Autodesk Inventor part; units mm, degrees
ref_plane "YZ Plane" through (0, 0, 0) normal (1, 0, 0) x (0, 1, 0)
ref_plane "XZ Plane" through (0, 0, 0) normal (0, 1, 0) x (-1, 0, 0)
ref_plane "XY Plane" through (0, 0, 0) normal (0, 0, 1) x (1, 0, 0)
sketch "Sketch1" plane through (0, 0, 0) normal (0, 0, 1) x (1, 0, 0)
  line L0 (11.7695, 33.9618) -> (11.7695, -67.6382)
  line L1 (100.6695, 33.9618) -> (100.6695, -67.6382)
  line L2 (18.1195, 40.3118) -> (94.3195, 40.3118)
  line L3 (24.4695, -80.3382) -> (87.9695, -80.3382)
  arc A0 (11.7695, -67.6382) -> (24.4695, -80.3382) centre (24.4695, -67.6382) ccw
  arc A1 (87.9695, -80.3382) -> (100.6695, -67.6382) centre (87.9695, -67.6382) ccw
  arc A2 (100.6695, 33.9618) -> (94.3195, 40.3118) centre (94.3195, 33.9618) ccw
  arc A3 (18.1195, 40.3118) -> (11.7695, 33.9618) centre (18.1195, 33.9618) ccw
  point P0 (0, 0)
  dimension "d0" = 12.7
  dimension "d1" = 6.35
  dimension "d2" = 120.65
  dimension "d3" = 88.9
extrude "Extrusion1" add sketch "Sketch1" along normal blind 4.7625
sketch "Sketch2" plane through (0, 0, 4.7625) normal (0, 0, 1) x (1, 0, 0)
  line L0 (11.7695, -67.6382) -> (11.7695, 33.9618)
  line L1 (100.6695, 33.9618) -> (100.6695, -67.6382)
  line L2 (18.1195, 40.3118) -> (94.3195, 40.3118)
  line L3 (17.7131, 34.3682) -> (94.7259, 34.3682)
  line L4 (94.7259, 34.3682) -> (94.7259, -29.6652)
  line L5 (94.7259, -29.6652) -> (17.7131, -29.6652)
  line L6 (17.7131, -29.6652) -> (17.7131, 34.3682)
  point P0 (0, 0)
  dimension "d6" = 5.9436
  dimension "d7" = 5.9436
  dimension "d8" = 5.9436
  dimension "d9" = 64.0334
  dimension "d54" = 77.0128
extrude "Extrusion2" cut sketch "Sketch2" against normal through all
sketch "Sketch3" plane through (0, 0, 4.7625) normal (0, 0, 1) x (1, 0, 0)
  line L0 (17.7131, -29.6652) -> (17.7131, 34.3682)
  line L1 (94.7259, 34.3682) -> (94.7259, -29.6652)
  line L2 (94.7259, -29.6652) -> (17.7131, -29.6652)
  line L3 (30.4131, -29.6652) -> (30.4131, -34.7452)
  line L4 (30.4131, -34.7452) -> (82.0259, -34.7452)
  line L5 (82.0259, -34.7452) -> (82.0259, -29.6652)
  point P0 (0, 0)
  dimension "d13" = 12.7
  dimension "d14" = 12.7
  dimension "d15" = 5.08
extrude "Extrusion3" cut sketch "Sketch3" against normal through all
sketch "Sketch4" plane through (0, 0, 4.7625) normal (0, 0, 1) x (1, 0, 0)
  line L0 (17.7131, -29.6652) -> (17.7131, 34.3682)
  line L1 (94.7259, 34.3682) -> (94.7259, -29.6652)
  line L2 (82.0259, -34.7452) -> (30.4131, -34.7452)
  arc A0 (11.7695, -67.6382) -> (24.4695, -80.3382) centre (24.4695, -67.6382) ccw
  line L3 (87.9695, -80.3382) -> (24.4695, -80.3382)
  arc A1 (87.9695, -80.3382) -> (100.6695, -67.6382) centre (87.9695, -67.6382) ccw
  line L4 (24.4695, -73.9882) -> (87.9695, -73.9882)
  line L5 (17.7131, -32.8402) -> (17.7131, -67.2318)
  line L6 (94.7259, -32.8402) -> (94.7259, -67.2318)
  arc A2 (17.7131, -67.2318) -> (24.4695, -73.9882) centre (24.4695, -67.2318) ccw
  arc A3 (87.9695, -73.9882) -> (94.7259, -67.2318) centre (87.9695, -67.2318) ccw
  line L7 (30.4131, -34.7452) -> (30.4131, -29.6652)
  line L8 (30.4131, -29.6652) -> (17.7131, -29.6652)
  line L9 (82.0259, -29.6652) -> (82.0259, -34.7452)
  line L10 (30.4131, -32.8402) -> (17.7131, -32.8402)
  line L11 (82.0259, -32.8402) -> (94.7259, -32.8402)
  point P0 (0, 0)
  dimension "d18" = 6.35
  dimension "d21" = 3.175
extrude "Extrusion4" cut sketch "Sketch4" against normal through all
sketch "Sketch6" plane through (0, 0, 4.7625) normal (0, 0, 1) x (1, 0, 0)
  line L0 (87.9695, -80.3382) -> (24.4695, -80.3382)
  circle A0 centre (37.1695, 37.1876) radius 1.27
  circle A1 centre (75.2695, 37.1876) radius 1.27
  circle A2 centre (37.1695, -77.214) radius 1.27
  circle A3 centre (75.2695, -77.214) radius 1.27
  circle A4 centre (14.8937, 21.2618) radius 1.27
  circle A5 centre (14.8937, -16.8382) radius 1.27
  circle A6 centre (97.5453, 21.2618) radius 1.27
  circle A7 centre (97.5453, -16.8382) radius 1.27
  line L1 (18.1195, 40.3118) -> (94.3195, 40.3118)
  line L2 (11.7695, -67.6382) -> (11.7695, 33.9618)
  line L3 (100.6695, 33.9618) -> (100.6695, -67.6382)
  point P0 (0, 0)
  dimension "d35" = 3.1242
  dimension "d36" = 3.1242
  dimension "d37" = 3.1242
  dimension "d38" = 3.1242
  dimension "d39" = 2.54
  dimension "d40" = 25.4
  dimension "d41" = 19.05
  dimension "d42" = 25.4
  dimension "d43" = 38.1
extrude "Extrusion5" cut sketch "Sketch6" against normal through all
sketch "Sketch7" plane through (0, 0, 4.7625) normal (0, 0, 1) x (1, 0, 0)
  circle A0 centre (97.5453, -16.8382) radius 1.27
  circle A1 centre (97.5453, 21.2618) radius 1.27
  circle A2 centre (14.8937, -16.8382) radius 1.27
  circle A3 centre (14.8937, 21.2618) radius 1.27
  circle A4 centre (75.2695, -77.214) radius 1.27
  circle A5 centre (37.1695, -77.214) radius 1.27
  circle A6 centre (75.2695, 37.1876) radius 1.27
  circle A7 centre (37.1695, 37.1876) radius 1.27
  line L0 (17.7131, -32.8402) -> (30.4131, -32.8402)
  line L1 (30.4131, -32.8402) -> (30.4131, -29.6652)
  line L2 (30.4131, -29.6652) -> (17.7131, -29.6652)
  line L3 (17.7131, -29.6652) -> (17.7131, 34.3682)
  line L4 (17.7131, 34.3682) -> (94.7259, 34.3682)
  line L5 (94.7259, 34.3682) -> (94.7259, -29.6652)
  line L6 (94.7259, -29.6652) -> (82.0259, -29.6652)
  line L7 (82.0259, -29.6652) -> (82.0259, -32.8402)
  line L8 (82.0259, -32.8402) -> (94.7259, -32.8402)
  line L9 (94.7259, -32.8402) -> (94.7259, -67.2318)
  arc A8 (87.9695, -73.9882) -> (94.7259, -67.2318) centre (87.9695, -67.2318) ccw
  line L10 (87.9695, -73.9882) -> (24.4695, -73.9882)
  arc A9 (17.7131, -67.2318) -> (24.4695, -73.9882) centre (24.4695, -67.2318) ccw
  line L11 (17.7131, -67.2318) -> (17.7131, -32.8402)
  arc A10 (18.1195, 40.3118) -> (11.7695, 33.9618) centre (18.1195, 33.9618) ccw
  line L12 (11.7695, -67.6382) -> (11.7695, 33.9618)
  arc A11 (11.7695, -67.6382) -> (24.4695, -80.3382) centre (24.4695, -67.6382) ccw
  line L13 (87.9695, -80.3382) -> (24.4695, -80.3382)
  arc A12 (87.9695, -80.3382) -> (100.6695, -67.6382) centre (87.9695, -67.6382) ccw
  line L14 (100.6695, 33.9618) -> (100.6695, -67.6382)
  arc A13 (100.6695, 33.9618) -> (94.3195, 40.3118) centre (94.3195, 33.9618) ccw
  line L15 (18.1195, 40.3118) -> (94.3195, 40.3118)
  line L16 (11.7695, -61.2882) -> (30.8195, -80.3382)
  line L17 (81.6195, -80.3382) -> (100.6695, -61.2882)
  point P0 (0, 0)
  dimension "d46" = 6.35
  dimension "d47" = 5.9436
  dimension "d48" = 82.9564
  dimension "d49" = 13.1064
  dimension "d50" = 12.7
  dimension "d51" = 19.05
  dimension "d52" = 19.05
  dimension "d53" = 69.85
properties part number "lcd_spacer"
Here's how the part is built. I have some questions about the finished solid (model axes, mm). A direction names the side the tool comes from. Give positions to 0.01 mm unless a question says otherwise; leave off trailing zeros. Order: outer loops, then holes, each group sorted by start corner. A loop starts at its lowest first (then second) coordinate and runs counter-clockwise, first axis right, second up. Notation, with made-up numbers: (22, -12.5) -> (30, -12.5) arc R24 ccw to (30, 11.5) -> close; hole circle Ø7 at (-2, -12). An arc over 180 degrees is marked (long way). Use CSV: the item, a comma, the result in double quotes. Start each with the question number.
Item 1: Suppose I cut it at C-C (x = 44.5). List the corners of the cut face in (y, z) for me.
Item 2: Thinking about a two-plate mould opening in Y: for faces 1 (the cylindrical face through (75.104, -75.955, 2.415)), 2 (the flat face through (56, -73.988, 2)), 3 (the flat face through (96, -20, 4.762)), 4 (the cylindrical face through (97.048, -76.519, 2.348)), which applies, pulls with the +Y half, pulls with the -Y half, needs draft (parallel to the pull), parting line crosses it, or undercut?
Item 3: Suppose I cut it at D-D (z = 2.6). Give the number of separate pieces and of enclosed holes in the cut face, and give its area (3 significant figures).
Item 4: Suppose I cut it at B-B (y = -13.5). List the corners of the cut face in (x, z) for me.
Item 5: If I drill on probe 1 along Y at (x, z) = (35, 3.7); probe 2 along X at (y, z) = (-19, 0.35); probe 3 along Y at (x, z) = (20, 2.75), over which ranges is the centre line in solid material (lowest first)? Write a range as [from, to].
Item 6: On a 3-axis mill with a long thin cutter (end or side, diameter ignored), from which of +Z, -Z, +X, -X, +Y, -Y can I reach the whole of each face in a straight line? I mean faces 5 (the flat face through (17.713, -50, 2)), 6 (the flat face through (96, -20, 0)). Say none if no direction works.
Item 7: Suppose I cut it at A-A (x = 86.5). List the corners of the cut face in (y, z) for me, and give its area (3 significant figures).
Answer block:
1,outline,"(-80.34, 0) -> (-73.99, 0) -> (-73.99, 4.76) -> (-80.34, 4.76) -> close; (34.37, 0) -> (40.31, 0) -> (40.31, 4.76) -> (34.37, 4.76) -> close"
2,face 1,"undercut"
2,face 2,"undercut"
2,face 3,"needs draft"
2,face 4,"pulls with the -Y half"
3,separate pieces,"1"
3,enclosed holes,"9"
3,area,"2,350 mm^2"
4,outline,"(11.77, 0) -> (17.71, 0) -> (17.71, 4.76) -> (11.77, 4.76) -> close; (94.73, 0) -> (100.67, 0) -> (100.67, 4.76) -> (94.73, 4.76) -> close"
5,probe 1,"y = [-80.34, -73.99], [34.37, 40.31]"
5,probe 2,"x = [11.77, 17.71], [94.73, 100.67]"
5,probe 3,"y = [-79.53, -72.3], [-32.84, -29.67], [34.37, 40.31]"
6,face 5,"+Z, -Z"
6,face 6,"-Z, +X, -X, +Y, -Y"
7,outline,"(-80.34, 0) -> (-73.99, 0) -> (-73.99, 4.76) -> (-80.34, 4.76) -> close; (-32.84, 0) -> (-29.67, 0) -> (-29.67, 4.76) -> (-32.84, 4.76) -> close; (34.37, 0) -> (40.31, 0) -> (40.31, 4.76) -> (34.37, 4.76) -> close"
7,area,"73.7 mm^2"
